Read the model definition and answer for the solid it produces. Units are mm, in the model's axes. A direction names the side the tool comes from. Coordinates: 2 decimals unless noted, no trailing zeros. Write each loop counter-clockwise with the first axis right and the second up, starting at its lowest first coordinate (ties: lowest second). Pieces come first, ordered by that corner, then holes. Notation, with made-up numbers: (51, 41.25) - (86, 41.25) arc R17 cw to (86, 61.25) - close; hole circle Ø8 at (2.25, -9.75). An arc over 180 degrees is marked (long way). Use a Markdown table: item, result.
from build123d import *

# Parameters (mm, degrees)
SKETCH1_W           = 21
SKETCH1_H           = 24
SKETCH1_W_2         = 19
SKETCH1_H_2         = 22
BOSS_EXTRUDE1_DEPTH = 8
SKETCH2_W           = 19
SKETCH2_H           = 22
BOSS_EXTRUDE2_DEPTH = 2
SKETCH3_R           = 2.1
CUT_EXTRUDE1_DEPTH  = 30


with BuildPart() as part:
    # Sketch1 → Boss-Extrude1 (new body)
    with BuildSketch(Plane.XY):
        Rectangle(SKETCH1_W, SKETCH1_H)
        Rectangle(SKETCH1_W_2, SKETCH1_H_2, mode=Mode.SUBTRACT)
    extrude(amount=BOSS_EXTRUDE1_DEPTH)

    # Sketch2 → Boss-Extrude2 (add)
    with BuildSketch(Plane(origin=(0, 0, 0), x_dir=(-1, 0, 0), z_dir=(0, 0, -1))):
        Rectangle(SKETCH2_W, SKETCH2_H)
    extrude(amount=-BOSS_EXTRUDE2_DEPTH)

    # Sketch3 → Cut-Extrude1 (cut)
    with BuildSketch(Plane.XZ.offset(12)):
        with Locations((0, 4)):
            Circle(SKETCH3_R)
    extrude(amount=-CUT_EXTRUDE1_DEPTH, mode=Mode.SUBTRACT)


solid = part.part
(1) The mould has two halves that part along Y. Classify faces 3 (the flat face through (-0.1, -11, 6.3)), 4 (the flat face through (0, 0, 0)), 5 (the flat face through (-2.5, -12, 3.9)), 6 (the flat face through (-2.5, 12, 3.9)): pulls with the +Y half, pulls with the -Y half, needs draft (parallel to the pull), parting line crosses it, or undercut.
Report:
| item | result |
|---|---|
| face 3 | undercut |
| face 4 | needs draft |
| face 5 | pulls with the -Y half |
| face 6 | pulls with the +Y half |
(2) A cutting plane is placed at B-B, the plane x = 0. Write down the section's boundary in (y, z), and give its area (3 significant figures).
Report:
| item | result |
|---|---|
| outline | (-12, 0) - (12, 0) - (12, 1.9) - (-12, 1.9) - close; (-12, 6.1) - (-11, 6.1) - (-11, 8) - (-12, 8) - close; (11, 6.1) - (12, 6.1) - (12, 8) - (11, 8) - close |
| area | 49.4 mm² |
(3) This flat-tipped pin is pushed along its axis until it touches: P1, Ø1.5, axis at x = -2.5, y = 8, coming from the +Z side. Where does it stop, or does it pass through?
Report:
| item | result |
|---|---|
| P1 | stops at z = 2 |
(4) A cutting plane is placed at D-D, the plane x = 8.25. Write down the section's boundary in (y, z).
Report:
| item | result |
|---|---|
| outline | (-12, 0) - (12, 0) - (12, 8) - (11, 8) - (11, 2) - (-11, 2) - (-11, 8) - (-12, 8) - close |
(5) A cutting plane is placed at A-A, the plane z = 4. Write down the section's boundary in (x, y), and give its area (3 significant figures).
Report:
| item | result |
|---|---|
| outline | (-10.5, -12) - (-2.1, -12) - (-2.1, -11) - (-9.5, -11) - (-9.5, 11) - (-2.1, 11) - (-2.1, 12) - (-10.5, 12) - close; (2.1, -12) - (10.5, -12) - (10.5, 12) - (2.1, 12) - (2.1, 11) - (9.5, 11) - (9.5, -11) - (2.1, -11) - close |
| area | 77.6 mm² |
(6) For faces 1 (the flat face through (-5, 0, 2)), 2 (the flat face through (-10, 0, 8)), determine the directions among +Z, -Z, +X, -X, +Y, -Y from which every point of the face is accessible in a straight line to the end or side of a thin tool.
Report:
| item | result |
|---|---|
| face 1 | +Z |
| face 2 | +Z, +X, -X, +Y, -Y |
(7) Straight lines are drawn through the part: L1, parallel to Y at x = -7, z = 6; L2, parallel to X at y = 4.75, z = 4.25; L3, parallel to Z at x = 7.75, y = 7.5. For each, find the intervals that lie inside material, in ascending order.
Report:
| item | result |
|---|---|
| L1 | y = -12 to -11, 11 to 12 |
| L2 | x = -10.5 to -9.5, 9.5 to 10.5 |
| L3 | z = 0 to 2 |
(8) A cutting plane is placed at C-C, the plane y = 4.5. Write down the section's boundary in (x, z), and give its area (3 significant figures).
Report:
| item | result |
|---|---|
| outline | (-10.5, 0) - (10.5, 0) - (10.5, 8) - (9.5, 8) - (9.5, 2) - (0.64, 2) arc R2.1 cw to (-0.64, 2) - (-9.5, 2) - (-9.5, 8) - (-10.5, 8) - close |
| area | 53.9 mm² |
